Geometry check sheet. Reference: drawing and pictorial views, mm from the part's lowest x, y, z. A direction names the side the tool comes from. Round coordinates to 2 decimals unless told otherwise and drop trailing zeros. Write each loop counter-clockwise with the first axis right and the second up, starting at its lowest first coordinate (ties: lowest second). Pieces come first, ordered by that corner, then holes.
Item 1: Section check B-B, the plane y = 30.5. Record the cut outline in (x, z).
Item 2: Section check A-A, the plane x = 10. Record the cut outline in (y, z), plus the area to 3 significant figures.
Item 3: Depth check by flat-ended pin: pin 1 (10 mm diameter, centred on x = 6.5, y = 28, fed in from +Z); pin 2 (12 mm diameter, centred on y = 32.5, z = 9.5, fed in from -X); pin 3 (3 mm diameter, centred on x = 8.5, z = 19.5, fed in from +Y); pin 4 (4 mm diameter, centred on x = 11.5, y = 29.5, fed in from +Z). Enter the tip coordinate at first touch or a pass-through.
Item 4: Set-up check for the marked faces 1, 2, 3, 4 and 5: record each of +Z, -Z, +X, -X, +Y, -Y from which the full face is reachable in a straight line by a thin tool's end or side.
Item 5: Section check C-C, the plane z = 10.25. Record the cut outline in (x, y).
Item 6: Section check D-D, the plane x = 7. Record the cut outline in (y, z).
Item 7: Release check for a two-part mould opening along X. For the marked faces 6, 7, 8 and 9 record: pulls with the +X half, pulls with the -X half, needs draft (parallel to the pull), parting line crosses it, or undercut.
Item 8: Material ranges on line 1 along Y through (x, z) = (10, 9.5); line 2 along Z through (x, y) = (10, 4.1); line 3 along Z through (x, y) = (15, 18.5), recorded low to high.
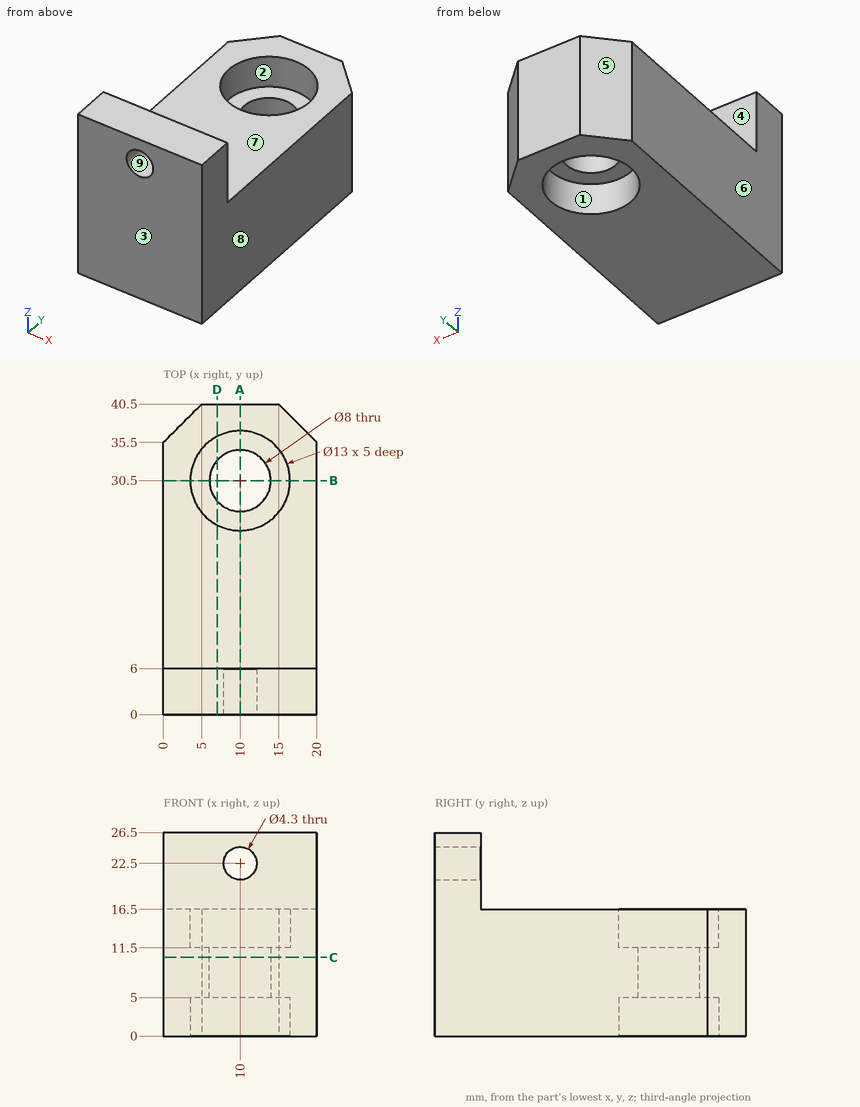
Values found:
1. outline: (0, 0) - (3.5, 0) - (3.5, 5) - (6, 5) - (6, 11.5) - (3.5, 11.5) - (3.5, 16.5) - (0, 16.5) - close; (14, 5) - (16.5, 5) - (16.5, 0) - (20, 0) - (20, 16.5) - (16.5, 16.5) - (16.5, 11.5) - (14, 11.5) - close
2. outline: (0, 0) - (24, 0) - (24, 5) - (26.5, 5) - (26.5, 11.5) - (24, 11.5) - (24, 16.5) - (6, 16.5) - (6, 20.35) - (0, 20.35) - close; (0, 24.65) - (6, 24.65) - (6, 26.5) - (0, 26.5) - close; (34.5, 5) - (37, 5) - (37, 0) - (40.5, 0) - (40.5, 16.5) - (37, 16.5) - (37, 11.5) - (34.5, 11.5) - close
2. area: 520 mm2
3. pin 1: stops at z = 16.5
3. pin 2: stops at x = 0
3. pin 3: stops at y = 6
3. pin 4: passes through
4. face 1: -Z
4. face 2: +Z
4. face 3: +Z, -Z, +X, -X, -Y
4. face 4: +Z, +X, -X, +Y
4. face 5: +Z, -Z, -X, +Y
5. outline: (0, 0) - (20, 0) - (20, 35.5) - (15, 40.5) - (5, 40.5) - (0, 35.5) - close; hole circle Ø8 at (10, 30.5)
6. outline: (0, 0) - (24.73, 0) - (24.73, 5) - (27.85, 5) - (27.85, 11.5) - (24.73, 11.5) - (24.73, 16.5) - (6, 16.5) - (6, 26.5) - (0, 26.5) - close; (33.15, 5) - (36.27, 5) - (36.27, 0) - (40.5, 0) - (40.5, 16.5) - (36.27, 16.5) - (36.27, 11.5) - (33.15, 11.5) - close
7. face 6: pulls with the -X half
7. face 7: needs draft
7. face 8: pulls with the +X half
7. face 9: undercut
8. line 1: y = 0 to 26.5, 34.5 to 40.5
8. line 2: z = 0 to 20.35, 24.65 to 26.5
8. line 3: z = 0 to 16.5
